The drawing under review shows one solid part. Ordinate dimensions are in mm from its lowest x, y, z. Give positions to 0.01 mm unless a question says otherwise; leave off trailing zeros. Write each loop counter-clockwise with the first axis right and the second up, starting at its lowest first coordinate (ties: lowest second). Pieces come first, ordered by that corner, then holes.
Q1. We need section B-B (y = 13). Write out the cut boundary in (x, z).
Q2. We need section A-A (x = 19.05). Write out the cut boundary in (y, z) (1 decimal), then the cut area to 3 significant figures.
Q3. For line 1 (X direction, y = 20, z = 11); line 2 (Z direction, x = 23.5, y = 27); line 3 (Y direction, x = 14.5, z = 25) (1 decimal), list the stretches that pass through material, from the lowest coordinate up.
Q4. Mouldability with a two-part tool opening along Y and no side actions: class the marked faces 1, 2 and 3 as released by +Y, released by -Y, zero draft, split by the parting line, or undercut.
Q5. Insertion check: P1, Ø3, axis at x = 28.5, y = 17, coming from the -Z side; P2, Ø10, axis at x = 8, z = 15, coming from the -Y side (1 decimal); P3, Ø8, axis at x = 12, z = 81, coming from the +Y side; P4, Ø6, axis at x = 32.5, z = 31, coming from the +Y side. Each pin has a flat end and moves straight along its axis. Give the tip position at first contact, or say it passes through.
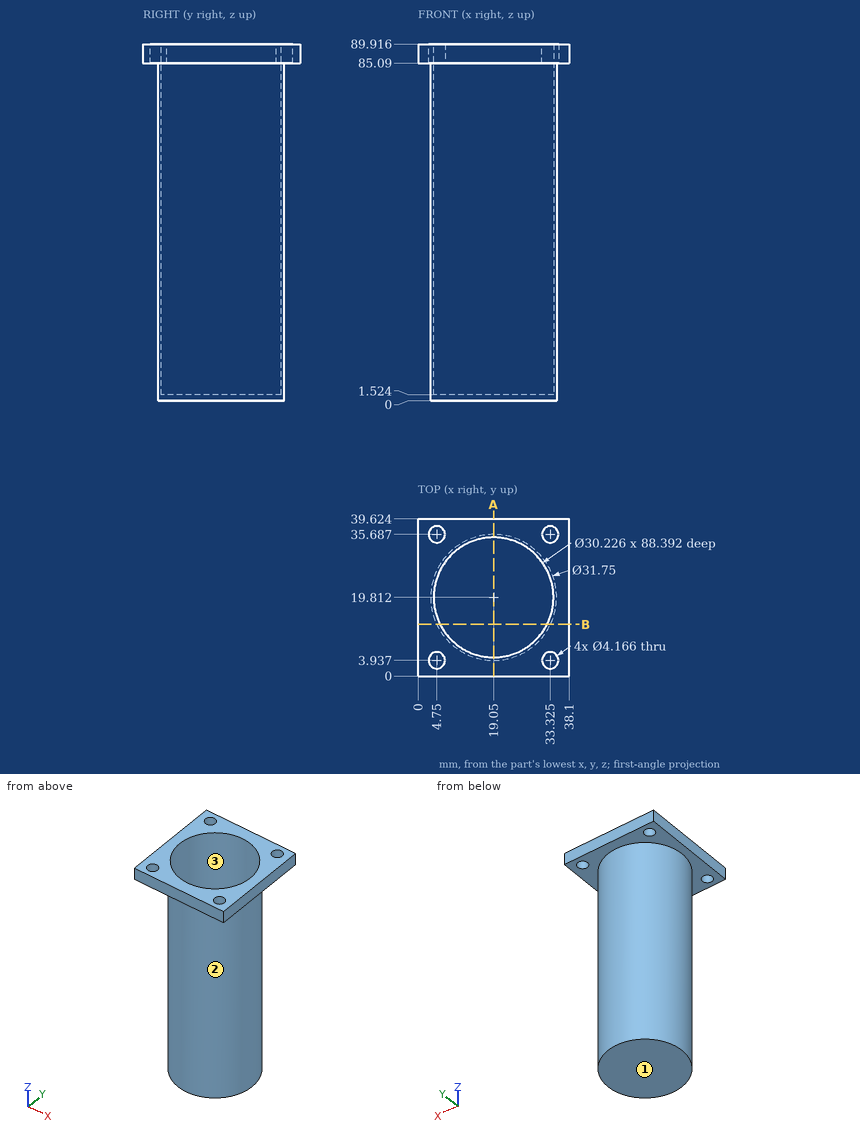
Computed:
1. outline: (0, 85.09) - (4.71, 85.09) - (4.71, 0) - (33.39, 0) - (33.39, 85.09) - (38.1, 85.09) - (38.1, 89.92) - (32.54, 89.92) - (32.54, 1.52) - (5.56, 1.52) - (5.56, 89.92) - (0, 89.92) - close
2. outline: (0, 85.1) - (3.9, 85.1) - (3.9, 0) - (35.7, 0) - (35.7, 85.1) - (39.6, 85.1) - (39.6, 89.9) - (34.9, 89.9) - (34.9, 1.5) - (4.7, 1.5) - (4.7, 89.9) - (0, 89.9) - close
2. area: 221 mm2
3. line 1: x = 3.18 to 3.94, 34.16 to 34.92
3. line 2: z = 0 to 1.52
3. line 3: y = 4.6 to 5.4, 34.2 to 35
4. face 1: zero draft
4. face 2: split by the parting line
4. face 3: undercut
5. P1: stops at z = 0
5. P2: stops at y = 5.1
5. P3: stops at y = 35.39
5. P4: stops at y = 31.76
